Could you check a few things on this drawing? It's one solid part, dimensions in mm from its lowest x, y, z. A direction names the side the tool comes from. Round coordinates to 2 decimals unless told otherwise and drop trailing zeros. Write each loop counter-clockwise with the first axis right and the second up, starting at its lowest first coordinate (ties: lowest second). Pieces come first, ordered by that corner, then holes. Notation, with made-up numbers: M 66.5,-11.75 L 118.5,-11.75 A23 ccw 118.5,15.25 Z; hole C 45.25,5 d5. An arc over 180 degrees is marked long. One line per question, with ' | ' between items. Start each with the question number.
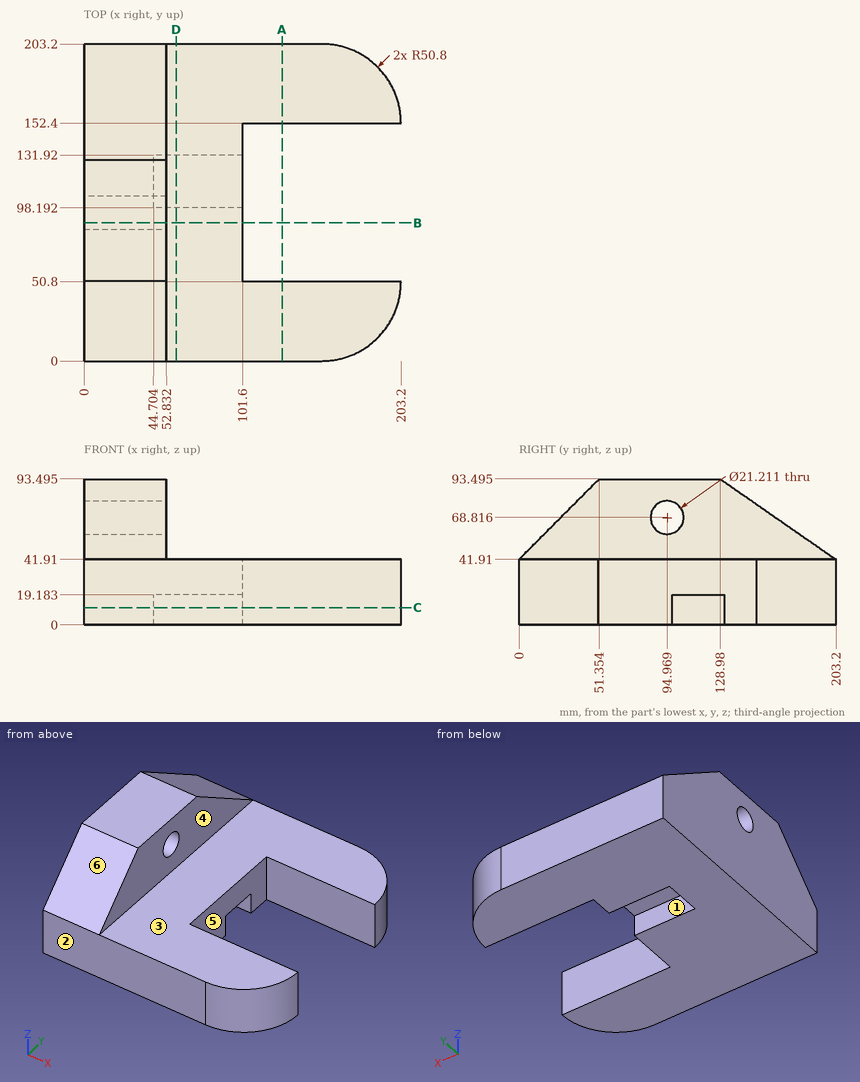
1. I need wall thicknesses on line 1 along Y through (x, z) = (105, 30); line 2 along X through (y, z) = (59.5, 86.5); line 3 along Z through (x, y) = (77, 164). Which ranges of each line are inside material? Lowest first, please. Write a range as from..to.
2. If we mould it in two halves opening along Y, with no side actions, what happens to the marked faces 1, 2 and 3? For each: released by +Y, released by -Y, zero draft, split by the parting line, or undercut.
3. Which directions (+Z, -Z, +X, -X, +Y, -Y) give clear straight access to the entire face, cutting with the end or side of a thin tool? Please do the marked faces 4, 5 and 6.
4. I'm going to push flat-ended pins straight in: P1, Ø6, axis at y = 123, z = 9, coming from the +X side; P2, Ø10, axis at y = 21, z = 39.5, coming from the +X side (1 decimal); P3, Ø3, axis at y = 117.5, z = 51.5, coming from the +X side; P4, Ø2, axis at x = 54.5, z = 68, coming from the +Y side. Where does each tip first touch, or does it pass through?
5. Suppose I cut it at D-D (x = 59). Write out the boundary of the cut face in (y, z).
6. Suppose I cut it at C-C (z = 11). Write out the boundary of the cut face in (x, y), and give its area (3 significant figures).
7. Suppose I cut it at A-A (x = 127). Write out the boundary of the cut face in (y, z), and give its area (3 significant figures).
8. Suppose I cut it at B-B (y = 88.5). Write out the boundary of the cut face in (x, z) (1 decimal).
Computed:
1) line 1: y = 0..50.8, 152.4..203.2 | line 2: x = 0..52.83 | line 3: z = 0..41.91
2) face 1: undercut | face 2: released by -Y | face 3: zero draft
3) face 4: +Z, +X, +Y, -Y | face 5: +Z, -Z, +X | face 6: +Z, +X, -X, -Y
4) P1: stops at x = 44.7 | P2: stops at x = 196.7 | P3: stops at x = 52.83 | P4: passes through
5) outline: M 0,0 L 98.19,0 L 98.19,19.18 L 131.92,19.18 L 131.92,0 L 203.2,0 L 203.2,41.91 L 0,41.91 Z
6) outline: M 0,0 L 152.4,0 A50.8 ccw 203.2,50.8 L 101.6,50.8 L 101.6,98.19 L 44.7,98.19 L 44.7,131.92 L 101.6,131.92 L 101.6,152.4 L 203.2,152.4 A50.8 ccw 152.4,203.2 L 0,203.2 Z | area: 27,900 mm²
7) outline: M 0,0 L 50.8,0 L 50.8,41.91 L 0,41.91 Z; M 152.4,0 L 203.2,0 L 203.2,41.91 L 152.4,41.91 Z | area: 4,260 mm²
8) outline: M 0,0 L 101.6,0 L 101.6,41.9 L 52.8,41.9 L 52.8,60.4 L 0,60.4 Z; M 0,77.2 L 52.8,77.2 L 52.8,93.5 L 0,93.5 Z
